```python
from build123d import *

# Parameters (mm, degrees)
SKETCH1_R           = 1.6
BOSS_EXTRUDE1_DEPTH = 5
BOSS_EXTRUDE2_START = -14
BOSS_EXTRUDE2_DEPTH = 5
CUT_EXTRUDE1_DEPTH  = 5
SKETCH2_4_W         = 7
SKETCH2_4_H         = 7.36
BOSS_EXTRUDE3_DEPTH = 14
BOSS_EXTRUDE4_START = -2
SKETCH3_R           = 1.6
BOSS_EXTRUDE4_DEPTH = 5
SKETCH3_3_R         = 1.6
CUT_EXTRUDE2_DEPTH  = 112.622599862
SKETCH3_4_W         = 7
SKETCH3_4_H         = 7.36
BOSS_EXTRUDE5_DEPTH = 3


with BuildPart() as part:
    # Sketch1 → Boss-Extrude1 (new body)
    with BuildSketch(Plane(origin=(0, 0, 0), x_dir=(1, 0, 0), z_dir=(0, 1, 0))):
        with BuildLine():
            Line((0, 3.68), (107, 3.68))
            ThreePointArc((107, 3.68), (110.68, 0), (107, -3.68))
            Line((107, -3.68), (0, -3.68))
            ThreePointArc((0, -3.68), (-3.68, 0), (0, 3.68))
        make_face()
        with Locations(Location((107, 0, 0), (0, 0, 270))):
            Circle(SKETCH1_R, mode=Mode.SUBTRACT)
        with BuildLine():
            Line((0, 1.6), (2, 1.6))
            ThreePointArc((2, 1.6), (3.6, 0), (2, -1.6))
            Line((2, -1.6), (0, -1.6))
            ThreePointArc((0, -1.6), (-1.6, 0), (0, 1.6))
        make_face(mode=Mode.SUBTRACT)
    extrude(amount=BOSS_EXTRUDE1_DEPTH)

    # Sketch2<3> → Cut-Extrude1 (cut)
    with BuildSketch(Plane.XZ):
        with BuildLine():
            ThreePointArc((0, 3.68), (-3.68, 0), (0, -3.68))
            Line((0, -3.68), (7.234142504, -3.68))
            Line((7.234142504, -3.68), (7.234142504, 3.68))
            Line((7.234142504, 3.68), (0, 3.68))
        make_face()
        with BuildLine():
            ThreePointArc((0, -1.6), (-1.6, 0), (0, 1.6))
            Line((0, 1.6), (2, 1.6))
            ThreePointArc((2, 1.6), (3.6, 0), (2, -1.6))
            Line((2, -1.6), (0, -1.6))
        make_face(mode=Mode.SUBTRACT)
    extrude(amount=-CUT_EXTRUDE1_DEPTH, mode=Mode.SUBTRACT)



with BuildPart() as body_2:
    # Sketch2 → Boss-Extrude2 (new body)
    with BuildSketch(Plane.XZ.offset(BOSS_EXTRUDE2_START)):
        with BuildLine():
            ThreePointArc((0, 3.68), (-3.68, 0), (0, -3.68))
            Line((0, -3.68), (7.234142504, -3.68))
            Line((7.234142504, -3.68), (7.234142504, 3.68))
            Line((7.234142504, 3.68), (0, 3.68))
        make_face()
        with BuildLine():
            ThreePointArc((0, -1.6), (-1.6, 0), (0, 1.6))
            Line((0, 1.6), (2, 1.6))
            ThreePointArc((2, 1.6), (3.6, 0), (2, -1.6))
            Line((2, -1.6), (0, -1.6))
        make_face(mode=Mode.SUBTRACT)
    extrude(amount=BOSS_EXTRUDE2_DEPTH)


with BuildPart() as part_1:
    add(part.part)

    add(body_2.part)  # Boss-Extrude3 merges body 2
    # Sketch2<4> → Boss-Extrude3 (add)
    with BuildSketch(Plane.XZ):
        with Locations((10.734142504, 0)):
            Rectangle(SKETCH2_4_W, SKETCH2_4_H)
    extrude(amount=-BOSS_EXTRUDE3_DEPTH)

    # Sketch3<3> → Cut-Extrude2 (cut, through all)
    # profile 1 of 2: a face of its own
    with BuildSketch(Plane.XZ):
        with BuildLine():
            ThreePointArc((110.68, 0), (109.602152955, 2.602152955), (107, 3.68))
            ThreePointArc((107, 3.68), (103.32, 0), (107, -3.68))
            ThreePointArc((107, -3.68), (109.602152955, -2.602152955), (110.68, 0))
        make_face()
        with Locations((107, 0)):
            Circle(SKETCH3_3_R, mode=Mode.SUBTRACT)
    # profile 2 of 2: a face of its own
    with BuildSketch(Plane.XZ):
        with BuildLine():
            ThreePointArc((107, -3.68), (103.32, 0), (107, 3.68))
            Line((107, 3.68), (50.58268169, 3.68))
            Line((50.58268169, 3.68), (50.58268169, -3.68))
            Line((50.58268169, -3.68), (107, -3.68))
        make_face()
    extrude(amount=-CUT_EXTRUDE2_DEPTH, mode=Mode.SUBTRACT)



with BuildPart() as body_2_2:
    # Sketch3 → Boss-Extrude4 (new body)
    # profile 1 of 2: a face of its own
    with BuildSketch(Plane.XZ.offset(BOSS_EXTRUDE4_START)):
        with BuildLine():
            ThreePointArc((107, -3.68), (103.32, 0), (107, 3.68))
            Line((107, 3.68), (50.58268169, 3.68))
            Line((50.58268169, 3.68), (50.58268169, -3.68))
            Line((50.58268169, -3.68), (107, -3.68))
        make_face()
    # profile 2 of 2: a face of its own
    with BuildSketch(Plane.XZ.offset(BOSS_EXTRUDE4_START)):
        with BuildLine():
            ThreePointArc((110.68, 0), (109.602152955, 2.602152955), (107, 3.68))
            ThreePointArc((107, 3.68), (103.32, 0), (107, -3.68))
            ThreePointArc((107, -3.68), (109.602152955, -2.602152955), (110.68, 0))
        make_face()
        with Locations((107, 0)):
            Circle(SKETCH3_R, mode=Mode.SUBTRACT)
    extrude(amount=BOSS_EXTRUDE4_DEPTH)


with BuildPart() as part_2:
    add(part_1.part)

    add(body_2_2.part)  # Boss-Extrude5 merges body 2 2
    # Sketch3<4> → Boss-Extrude5 (add)
    with BuildSketch(Plane.XZ):
        with Locations((47.08268169, 0)):
            Rectangle(SKETCH3_4_W, SKETCH3_4_H)
    extrude(amount=BOSS_EXTRUDE5_DEPTH)


solid = part_2.part
```
Design review of the part built by this model. Coordinates are the model's own, in mm. A direction names the side the tool comes from. Give positions to 0.01 mm unless a question says otherwise; leave off trailing zeros. Write each loop counter-clockwise with the first axis right and the second up, starting at its lowest first coordinate (ties: lowest second). Pieces come first, ordered by that corner, then holes. Notation, with made-up numbers: (65.5, -4) - (124.5, -4) arc R9 ccw to (124.5, 5) - close; hole circle Ø1 at (75, -16). An arc over 180 degrees is marked (long way). Return JSON: item names as keys, results as strings. Group by question number.
(1) Insertion check: pin 1 (2 mm diameter, centred on y = 11.5, z = -1, fed in from +X); pin 2 (2.5 mm diameter, centred on y = 3.5, z = -1.5, fed in from +X); pin 3 (3.5 mm diameter, centred on y = 3, z = 0.5, fed in from -X); pin 4 (3 mm diameter, centred on x = 39, y = -0.5, fed in from +Z). Each pin has a flat end and moves straight along its axis. Give the tip position at first contact, or say it passes through.
(2) Machinability: for faces 5 (the flat face through (33, 5, 0)), 6 (the flat face through (7, 14, 0)), 7 (the flat face through (26, 0, 0)), 8 (the flat face through (1, 12, -1.6)), which of the approach directions +Z, -Z, +X, -X, +Y, -Y give a long, thin tool a straight path to every point of the face, cutting with its end or side? Answer none if there is none.
(3) We need section B-B, the plane x = 45. Give the boundary of the cut face in (y, z).
(4) To check wall thickness, follow probe 1 along Z at (x, y) = (107, -0.75); probe 2 along Y at (x, z) = (94, 1); probe 3 along Y at (x, z) = (31.5, 2.75). State the ranges of each line that lie inside material, in increasing order.
(5) Mouldability with a two-part tool opening along Z and no side actions: class faces 1 (the cylindrical face through (-1.6, 11.5, 0)), 2 (the flat face through (43.583, -1, 0)), 3 (the cylindrical face through (3.6, 11.5, 0)), 4 (the flat face through (49, 2, -3.68)) as +Z half, -Z half, draft (parallel to the pull), parting line (faces both ways), or undercut.
(6) We need section A-A, the plane x = 67. Give the boundary of the cut face in (y, z), then the cut area to 3 significant figures.
Reported:
{
 "1": {"pin 1": "stops at x = 14.23", "pin 2": "stops at x = 50.58", "pin 3": "stops at x = 7.23", "pin 4": "stops at z = 3.68"},
 "2": {"face 5": "+Z, -Z, +X, +Y", "face 6": "+Z, -Z, +X, -X, +Y", "face 7": "+Z, -Z, -X, -Y", "face 8": "+Y, -Y"},
 "3": {"outline": "(-3, -3.68) - (5, -3.68) - (5, 3.68) - (-3, 3.68) - close"},
 "4": {"probe 1": "z = -3.68 to -1.6, 1.6 to 3.68", "probe 2": "y = -3 to 2", "probe 3": "y = 0 to 5"},
 "5": {"face 1": "undercut", "face 2": "draft", "face 3": "undercut", "face 4": "-Z half"},
 "6": {"outline": "(-3, -3.68) - (2, -3.68) - (2, 3.68) - (-3, 3.68) - close", "area": "36.8 mm2"}
}
